Read the model definition and answer for the solid it produces. Units are mm, in the model's axes. Face numbers are marked on the shaded views. A direction names the side the tool comes from. Give positions to 0.01 mm unless a question says otherwise; leave off trailing zeros. Loops run counter-clockwise (first coordinate to the right, second up) from the corner with the lowest first, then second, coordinate; pieces in that order, holes last. Notation, with made-up numbers: (-2.5, 3.25) - (51.5, 3.25) arc R22 ccw to (51.5, 31.25) - close; hole circle Ø3 at (17.5, 26). An arc over 180 degrees is marked (long way). Use a Markdown table: item, result. Add a question column.
Item 1: Which of the six approach directions +Z, -Z, +X, -X, +Y, -Y give full straight-line access (tool end or side, diameter ignored) to the marked faces 4 and 5?
Item 2: A cutting plane is placed at A-A (y = 75). Determine the outline of the cut face in (x, z), plus the area to 3 significant figures.
Item 3: For a pull along X with two mould halves and no side action, classify the marked faces 1, 2 and 3 as +X half, -X half, draft (parallel to the pull), parting line (faces both ways), or undercut.
Item 4: A cutting plane is placed at D-D (z = 10.5). Determine the outline of the cut face in (x, y), plus the area to 3 significant figures.
Item 5: A cutting plane is placed at B-B (z = 93). Determine the outline of the cut face in (x, y), plus the area to 3 significant figures.
Item 6: A cutting plane is placed at C-C (x = 70). Determine the outline of the cut face in (y, z), plus the area to 3 significant figures.
Item 7: Consider probe 1 along Y at (x, z) = (70, 4.65); probe 2 along Y at (x, z) = (15, 129.5); probe 3 along X at (y, z) = (105, 15). Determine where each line is inside the solid, lowest interval first. Write a range as [from, to].
Item 8: Each of these flat-tipped pins is pushed along its axis until it touches: P1, Ø1.5, axis at x = 88, y = 2.5, coming from the +Z side; P2, Ø6, axis at x = 85, y = 130.5, coming from the +Z side. Where does it stop, or does it pass through?
from build123d import *

# Parameters (mm, degrees)
ESBO_O1_W                                    = 140
ESBO_O1_H                                    = 150
RESSALTO_EXTRUS_O1_DEPTH                     = 6
ESBO_O2_W                                    = 140
ESBO_O2_H                                    = 150
ESBO_O2_W_2                                  = 130
ESBO_O2_H_2                                  = 140
RESSALTO_EXTRUS_O2_DEPTH                     = 150
ESBO_O3_W                                    = 80.487326646
ESBO_O3_H                                    = 259.40979835
CORTE_EXTRUS_O1_DEPTH                        = 150
ESBO_O4_W                                    = 259.40979835
ESBO_O4_H                                    = 111.824801178
CORTE_EXTRUS_O2_DEPTH                        = 150
ESCAREADO_PARA_PARAFUSO_COM_CABE_A_E_2_COUNT = 2
ESCAREADO_PARA_PARAFUSO_COM_CABE_A_E_2_PITCH = 94.314867898
ESCAREADO_PARA_PARAFUSO_COM_CABE_A_E_3_COUNT = 2
ESCAREADO_PARA_PARAFUSO_COM_CABE_A_E_3_PITCH = 104.661646655
ESCAREADO_PARA_PARAFUSO_COM_CABE_A_E_4_COUNT = 2
ESCAREADO_PARA_PARAFUSO_COM_CABE_A_E_4_PITCH = 140.887737533
ESBO_O11_W                                   = 80.487326646
ESBO_O11_H                                   = 5
RESSALTO_EXTRUS_O5_DEPTH                     = 15
ESBO_O12_W                                   = 63.61017092
ESBO_O12_H                                   = 5.135500038
CORTE_EXTRUS_O3_DEPTH                        = 219
ESBO_O13_R                                   = 56.69336486
CORTE_EXTRUS_O4_DEPTH                        = 10


with BuildPart() as part:
    # Esboço1 → Ressalto-extrusão1 (new body)
    with BuildSketch(Plane.XY):
        with Locations((70, 75)):
            Rectangle(ESBO_O1_W, ESBO_O1_H)
    extrude(amount=RESSALTO_EXTRUS_O1_DEPTH)

    # Esboço2 → Ressalto-extrusão2 (add)
    with BuildSketch(Plane.XY.offset(6)):
        with Locations((70, 75)):
            Rectangle(ESBO_O2_W, ESBO_O2_H)
        with Locations((70, 75)):
            Rectangle(ESBO_O2_W_2, ESBO_O2_H_2, mode=Mode.SUBTRACT)
    extrude(amount=RESSALTO_EXTRUS_O2_DEPTH)

    # Esboço3 → Corte-extrusão1 (cut)
    with BuildSketch(Plane.XZ):
        with Locations((70, 156)):
            Rectangle(ESBO_O3_W, ESBO_O3_H)
    extrude(amount=-CORTE_EXTRUS_O1_DEPTH, mode=Mode.SUBTRACT)

    # Esboço4 → Corte-extrusão2 (cut)
    with BuildSketch(Plane.ZY):
        with Locations((156, 75)):
            Rectangle(ESBO_O4_W, ESBO_O4_H)
    extrude(amount=-CORTE_EXTRUS_O2_DEPTH, mode=Mode.SUBTRACT)

    # Esboço6 → Escareado para parafuso com cabeça escareada elevada de M61 (revolve, cut)
    with BuildSketch(Plane(origin=(22.842566051, 127.330823328, 6), x_dir=(0, -1, 0), z_dir=(1, 0, 0))):
        Polygon((0, 0), (0, 6), (3.5, 6), (3.5, 2.8), (6.3, 0), align=None)
    escareado_para_parafuso_com_cabe_a_escar = revolve(axis=Axis((22.842566051, 127.330823328, 12.35), (0, 0, -1)), mode=Mode.SUBTRACT)

    # Escareado para parafuso com cabe_a e 2: Escareado para parafuso com cabeça escareada elevada de M61 ×2
    with Locations(*[(i * ESCAREADO_PARA_PARAFUSO_COM_CABE_A_E_2_PITCH, 0, 0) for i in range(1, ESCAREADO_PARA_PARAFUSO_COM_CABE_A_E_2_COUNT)]):
        add(escareado_para_parafuso_com_cabe_a_escar, mode=Mode.SUBTRACT)

    # Escareado para parafuso com cabe_a e 3: Escareado para parafuso com cabeça escareada elevada de M61 ×2
    with Locations(*[(0, -i * ESCAREADO_PARA_PARAFUSO_COM_CABE_A_E_3_PITCH, 0) for i in range(1, ESCAREADO_PARA_PARAFUSO_COM_CABE_A_E_3_COUNT)]):
        add(escareado_para_parafuso_com_cabe_a_escar, mode=Mode.SUBTRACT)

    # Escareado para parafuso com cabe_a e 4: Escareado para parafuso com cabeça escareada elevada de M61 ×2
    with Locations(*[Vector(0.6694327664681964, -0.7428726480216763, 0) * (i * ESCAREADO_PARA_PARAFUSO_COM_CABE_A_E_4_PITCH) for i in range(1, ESCAREADO_PARA_PARAFUSO_COM_CABE_A_E_4_COUNT)]):
        add(escareado_para_parafuso_com_cabe_a_escar, mode=Mode.SUBTRACT)

    # Esboço11 → Ressalto-extrusão5 (add)
    with BuildSketch(Plane.XY.offset(26.295100825)):
        with Locations((70, 147.5)):
            Rectangle(ESBO_O11_W, ESBO_O11_H)
        with Locations((70, 2.5)):
            Rectangle(ESBO_O11_W, ESBO_O11_H)
    extrude(amount=RESSALTO_EXTRUS_O5_DEPTH)

    # Esboço12 → Corte-extrusão3 (cut)
    with BuildSketch(Plane.XZ):
        with Locations((70, 28.296802645)):
            Rectangle(ESBO_O12_W, ESBO_O12_H)
    extrude(amount=-CORTE_EXTRUS_O3_DEPTH, mode=Mode.SUBTRACT)

    # Esboço13 → Corte-extrusão4 (cut)
    with BuildSketch(Plane.XY.offset(6)):
        with Locations((70, 75)):
            Circle(ESBO_O13_R)
    extrude(amount=-CORTE_EXTRUS_O4_DEPTH, mode=Mode.SUBTRACT)


solid = part.part
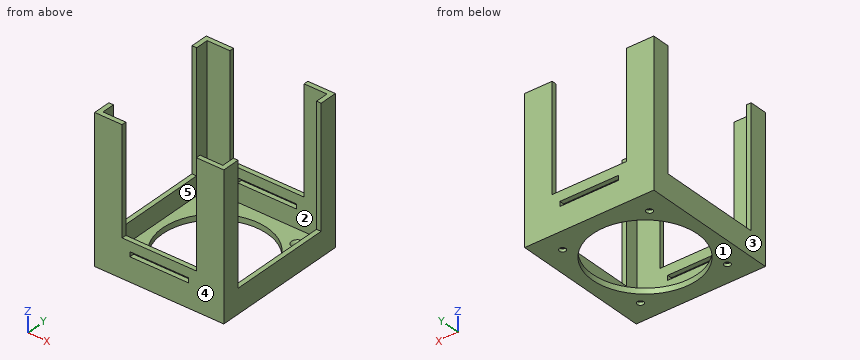
Geometry says:
| question | item | result |
|---|---|---|
| 1 | face 4 | +Z, -Z, +X, -X, -Y |
| 1 | face 5 | +Z |
| 2 | outline | (0, 0) - (13.31, 0) - (13.31, 6) - (5, 6) - (5, 26.3) - (0, 26.3) - close; (126.69, 0) - (140, 0) - (140, 26.3) - (135, 26.3) - (135, 6) - (126.69, 6) - close |
| 2 | area | 363 mm² |
| 3 | face 1 | draft |
| 3 | face 2 | undercut |
| 3 | face 3 | -X half |
| 4 | outline | (0, 0) - (140, 0) - (140, 150) - (0, 150) - close; hole (5, 5) - (135, 5) - (135, 145) - (5, 145) - close |
| 4 | area | 2,800 mm² |
| 5 | outline | (0, 0) - (29.76, 0) - (29.76, 5) - (5, 5) - (5, 19.09) - (0, 19.09) - close; (0, 130.91) - (5, 130.91) - (5, 145) - (29.76, 145) - (29.76, 150) - (0, 150) - close; (110.24, 0) - (140, 0) - (140, 19.09) - (135, 19.09) - (135, 5) - (110.24, 5) - close; (110.24, 145) - (135, 145) - (135, 130.91) - (140, 130.91) - (140, 150) - (110.24, 150) - close |
| 5 | area | 877 mm² |
| 6 | outline | (0, 0) - (18.31, 0) - (18.31, 6) - (5, 6) - (5, 25.73) - (0, 25.73) - close; (0, 30.86) - (5, 30.86) - (5, 41.3) - (0, 41.3) - close; (131.69, 0) - (150, 0) - (150, 25.73) - (145, 25.73) - (145, 6) - (131.69, 6) - close; (145, 30.86) - (150, 30.86) - (150, 41.3) - (145, 41.3) - close |
| 6 | area | 521 mm² |
| 7 | probe 1 | [0, 18.31], [131.69, 150] |
| 7 | probe 2 | [0, 5], [145, 150] |
| 7 | probe 3 | [0, 5], [135, 140] |
| 8 | P1 | z = 41.3 |
| 8 | P2 | z = 6 |
